Here's how the part is built. I have some questions about the finished solid (model axes, mm). A direction names the side the tool comes from. Give positions to 0.01 mm unless a question says otherwise; leave off trailing zeros. Loops run counter-clockwise (first coordinate to the right, second up) from the corner with the lowest first, then second, coordinate; pieces in that order, holes last. Notation, with made-up numbers: (43, 19) - (98, 19) arc R21 cw to (98, 25) - close; hole circle Ø4 at (-11.5, 47.5). An arc over 180 degrees is marked (long way). Use one line per item in the form item = value.
from build123d import *

# Parameters (mm, degrees)
F0_W     = 150
F0_H     = 92
F0_R     = 6
F0_R_2   = 3.5
F0_R_3   = 10
F0_R_4   = 8
F1_DEPTH = 2.5
F2_W     = 150
F2_H     = 92
F2_R     = 6
F2_R_2   = 10
F2_R_3   = 8
F3_DEPTH = 2.5
F4_W     = 150
F4_H     = 92
F5_DEPTH = 40
F6_R     = 5


with BuildPart() as f1:
    # F0 (on Top) → F1 (new body)
    with BuildSketch(Plane.XY):
        with Locations((75, 46)):
            Rectangle(F0_W, F0_H)
        with Locations((21.5, 23)):
            Circle(F0_R, mode=Mode.SUBTRACT)
        with Locations((43, 23)):
            Circle(F0_R, mode=Mode.SUBTRACT)
        with Locations((64.5, 23)):
            Circle(F0_R, mode=Mode.SUBTRACT)
        with Locations((85.5, 23)):
            Circle(F0_R, mode=Mode.SUBTRACT)
        with Locations((107, 23)):
            Circle(F0_R, mode=Mode.SUBTRACT)
        with Locations((101.5, 43)):
            Circle(F0_R_2, mode=Mode.SUBTRACT)
        with Locations((128.5, 23)):
            Circle(F0_R, mode=Mode.SUBTRACT)
        with Locations((133.5, 43)):
            Circle(F0_R_2, mode=Mode.SUBTRACT)
        with Locations((25, 59)):
            Circle(F0_R_3, mode=Mode.SUBTRACT)
        with Locations((50, 59)):
            Circle(F0_R_3, mode=Mode.SUBTRACT)
        with Locations((75, 59)):
            Circle(F0_R_3, mode=Mode.SUBTRACT)
        with Locations((117.5, 59)):
            Circle(F0_R_4, mode=Mode.SUBTRACT)
        with Locations((101.5, 75)):
            Circle(F0_R_2, mode=Mode.SUBTRACT)
        with Locations((133.5, 75)):
            Circle(F0_R_2, mode=Mode.SUBTRACT)
    extrude(amount=F1_DEPTH)

    # F2 (on face) → F3 (join)
    with BuildSketch(Plane.XY):
        with Locations((75, 46)):
            Rectangle(F2_W, F2_H)
        with Locations((21.5, 23)):
            Circle(F2_R, mode=Mode.SUBTRACT)
        with Locations((43, 23)):
            Circle(F2_R, mode=Mode.SUBTRACT)
        with Locations((64.5, 23)):
            Circle(F2_R, mode=Mode.SUBTRACT)
        with Locations((85.5, 23)):
            Circle(F2_R, mode=Mode.SUBTRACT)
        with Locations((107, 23)):
            Circle(F2_R, mode=Mode.SUBTRACT)
        with Locations((101.5, 43)):
            Circle(F2_R, mode=Mode.SUBTRACT)
        with Locations((128.5, 23)):
            Circle(F2_R, mode=Mode.SUBTRACT)
        with Locations((133.5, 43)):
            Circle(F2_R, mode=Mode.SUBTRACT)
        with Locations((25, 59)):
            Circle(F2_R_2, mode=Mode.SUBTRACT)
        with Locations((50, 59)):
            Circle(F2_R_2, mode=Mode.SUBTRACT)
        with Locations((75, 59)):
            Circle(F2_R_2, mode=Mode.SUBTRACT)
        with Locations((117.5, 59)):
            Circle(F2_R_3, mode=Mode.SUBTRACT)
        with Locations((101.5, 75)):
            Circle(F2_R, mode=Mode.SUBTRACT)
        with Locations((133.5, 75)):
            Circle(F2_R, mode=Mode.SUBTRACT)
    extrude(amount=-F3_DEPTH)

    # F4 (on face) → F5 (join)
    with BuildSketch(Plane(origin=(0, 0, -2.5), x_dir=(1, 0, 0), z_dir=(0, 0, -1))):
        with Locations((75, -46)):
            Rectangle(F4_W, F4_H)
        with BuildLine():
            ThreePointArc((1.5, -6.5), (2.964466, -2.964466), (6.5, -1.5))
            Line((6.5, -1.5), (143.5, -1.5))
            ThreePointArc((143.5, -1.5), (147.035534, -2.964466), (148.5, -6.5))
            Line((148.5, -6.5), (148.5, -85.5))
            ThreePointArc((148.5, -85.5), (147.035534, -89.035534), (143.5, -90.5))
            Line((143.5, -90.5), (6.5, -90.5))
            ThreePointArc((6.5, -90.5), (2.964466, -89.035534), (1.5, -85.5))
            Line((1.5, -85.5), (1.5, -6.5))
        make_face(mode=Mode.SUBTRACT)
    extrude(amount=F5_DEPTH)

    # F6
    f6_edges = [f1.edges().sort_by_distance(p)[0] for p in [
        (75, 0, 2.5),
        (150, 0, -20),
        (150, 46, 2.5),
        (150, 92, -20),
        (75, 92, 2.5),
        (0, 46, 2.5),
        (0, 92, -20),
        (0, 0, -20),
    ]]
    fillet(f6_edges, radius=F6_R)


solid = f1.part
(1) If we section it at B-B (y = 75): List the corners of the cut face in (x, z) for me, plus the area to 3 significant figures.
Geometry says:
outline = (0, -42.5) - (1.5, -42.5) - (1.5, -2.5) - (95.5, -2.5) - (95.5, 0) - (98, 0) - (98, 2.5) - (5, 2.5) arc R5 ccw to (0, -2.5) - close; (105, 0) - (107.5, 0) - (107.5, -2.5) - (127.5, -2.5) - (127.5, 0) - (130, 0) - (130, 2.5) - (105, 2.5) - close; (137, 0) - (139.5, 0) - (139.5, -2.5) - (148.5, -2.5) - (148.5, -42.5) - (150, -42.5) - (150, -2.5) arc R5 ccw to (145, 2.5) - (137, 2.5) - close
area = 764 mm²
(2) Thinking about a two-plate mould opening in Y: for faces 3 (the flat face through (74, 92, -22)), 4 (the flat face through (150, 47, -22)), 5 (the cylindrical face through (97.08, 79.06, -1.23)), 6 (the flat face through (74, 0, -22)), which applies, pulls with the +Y half, pulls with the -Y half, needs draft (parallel to the pull), parting line crosses it, or undercut?
Geometry says:
face_3 = pulls with the +Y half
face_4 = needs draft
face_5 = undercut
face_6 = pulls with the -Y half
(3) If I drill on probe 1 along X at (y, z) = (36.5, -20); probe 2 along Y at (x, z) = (117, -3.5); probe 3 along Y at (x, z) = (101.5, 1.45), over which ranges is the centre line in solid material (lowest first)?
Geometry says:
probe_1 = 0 to 1.5, 148.5 to 150
probe_2 = 0 to 1.5, 90.5 to 92
probe_3 = 1.93 to 20.6, 25.4 to 39.5, 46.5 to 71.5, 78.5 to 90.07
(4) For P1, Ø7, axis at x = 64.5, y = 23, coming from the -Z side; P2, Ø19, axis at x = 101.5, y = 75, coming from the -Z side; P3, Ø11, axis at x = 101.5, y = 43, coming from the -Z side, each with a flat end and sliding along its axis, tell me the tip position at first contact or that it passes through.
Geometry says:
P1 = through
P2 = -2.5
P3 = 0
(5) If we section it at A-A (y = 59): List the corners of the cut face in (x, z) for me, plus the area to 3 significant figures.
Geometry says:
outline = (0, -42.5) - (1.5, -42.5) - (1.5, -2.5) - (15, -2.5) - (15, 2.5) - (5, 2.5) arc R5 ccw to (0, -2.5) - close; (35, -2.5) - (40, -2.5) - (40, 2.5) - (35, 2.5) - close; (60, -2.5) - (65, -2.5) - (65, 2.5) - (60, 2.5) - close; (85, -2.5) - (109.5, -2.5) - (109.5, 2.5) - (85, 2.5) - close; (125.5, -2.5) - (148.5, -2.5) - (148.5, -42.5) - (150, -42.5) - (150, -2.5) arc R5 ccw to (145, 2.5) - (125.5, 2.5) - close
area = 479 mm²
(6) If we section it at C-C (z = -38): List the corners of the cut face in (x, y) for me.
Geometry says:
outline = (0, 5) arc R5 ccw to (5, 0) - (145, 0) arc R5 ccw to (150, 5) - (150, 87) arc R5 ccw to (145, 92) - (5, 92) arc R5 ccw to (0, 87) - close; hole (1.5, 6.5) arc R5 ccw to (6.5, 1.5) - (143.5, 1.5) arc R5 ccw to (148.5, 6.5) - (148.5, 85.5) arc R5 ccw to (143.5, 90.5) - (6.5, 90.5) arc R5 ccw to (1.5, 85.5) - close
(7) For faces 1 (the cylindrical face through (103.38, 45.95, 1.23)), 2 (the flat face through (74, 47, -2.5)), which set-ups out of +Z, -Z, +X, -X, +Y, -Y let a thin tool reach every point of the face, with its end or its side?
Geometry says:
face_1 = +Z, -Z
face_2 = -Z
(8) If we section it at D-D (x = 117.5): List the corners of the cut face in (y, z) for me.
Geometry says:
outline = (0, -42.5) - (1.5, -42.5) - (1.5, -2.5) - (51, -2.5) - (51, 2.5) - (5, 2.5) arc R5 ccw to (0, -2.5) - close; (67, -2.5) - (90.5, -2.5) - (90.5, -42.5) - (92, -42.5) - (92, -2.5) arc R5 ccw to (87, 2.5) - (67, 2.5) - close
